from build123d import *

# Parameters (mm, degrees)
F0_R     = 1.4224
F1_DEPTH = 2.9718


with BuildPart() as f1:
    # F0 (on Front) → F1 (new body)
    with BuildSketch(Plane.XZ):
        Polygon((0, 25.4), (0, 0), (50.8, 0), (50.8, 11.2776), (45.72, 11.2776), (45.72, 8.1026), (42.545, 8.1026), (42.545, 11.2776), (36.957, 11.2776), (36.957, 14.1224), (42.545, 14.1224), (42.545, 17.2974), (45.72, 17.2974), (45.72, 14.1224), (50.8, 14.1224), (50.8, 25.4), align=None)
        with Locations((1.4859, 12.7)):
            Circle(F0_R, mode=Mode.SUBTRACT)
    extrude(amount=F1_DEPTH)


solid = f1.part
Build history of the part. All positions in model axes, mm. A direction names the side the tool comes from. Coordinates: 2 decimals unless noted, no trailing zeros. Order: outer loops, then holes, each group sorted by start corner. A loop starts at its lowest first (then second) coordinate and runs counter-clockwise, first axis right, second up. Notation, with made-up numbers: (27, -16.5) -> (66, -16.5) arc R34 cw to (66, 21.5) -> close; hole circle Ø11 at (47, 3.5). An arc over 180 degrees is marked (long way). One line per item, written item: value.
(1) Slice it at C-C, the plane z = 10.75. List the corners of the cut face in (x, y) (3 decimals), plus the area to 3 significant figures.
Checked values:
outline: (0, -2.972) -> (42.545, -2.972) -> (42.545, 0) -> (0, 0) -> close; (45.72, -2.972) -> (50.8, -2.972) -> (50.8, 0) -> (45.72, 0) -> close
area: 142 mm2
(2) Mould opens along Z. For faces 4 (the flat face through (25, -2.972, 13)), 5 (the flat face through (26, -1, 25.4)), 6 (the flat face through (48, -1, 11.278)) say: pulls with the +Z half, pulls with the -Z half, needs draft (parallel to the pull), parting line crosses it, or undercut.
Checked values:
face 4: needs draft
face 5: pulls with the +Z half
face 6: undercut
(3) Slice it at A-A, the plane y = -2.5. List the corners of the cut face in (x, z) (3 decimals).
Checked values:
outline: (0, 0) -> (50.8, 0) -> (50.8, 11.278) -> (45.72, 11.278) -> (45.72, 8.103) -> (42.545, 8.103) -> (42.545, 11.278) -> (36.957, 11.278) -> (36.957, 14.122) -> (42.545, 14.122) -> (42.545, 17.297) -> (45.72, 17.297) -> (45.72, 14.122) -> (50.8, 14.122) -> (50.8, 25.4) -> (0, 25.4) -> close; hole circle Ø2.845 at (1.486, 12.7)
(4) Slice it at B-B, the plane x = 39. List the corners of the cut face in (y, z), plus the area to 3 significant figures.
Checked values:
outline: (-2.97, 0) -> (0, 0) -> (0, 11.28) -> (-2.97, 11.28) -> close; (-2.97, 14.12) -> (0, 14.12) -> (0, 25.4) -> (-2.97, 25.4) -> close
area: 67.0 mm2
(5) Tool access for faces 1 (the flat face through (36.957, -1, 13)), 2 (the flat face through (50.8, -1, 6)), 3 (the flat face through (45.72, -1, 10)): list every direction of +Z, -Z, +X, -X, +Y, -Y with a clear straight run to the whole face (end or side of a thin tool).
Checked values:
face 1: +X, +Y, -Y
face 2: +Z, -Z, +X, +Y, -Y
face 3: +Y, -Y
(6) Probe line 1 (Z direction, x = 46, y = -1.1); line 2 (Z direction, x = 45.5, y = -1.05); line 3 (X direction, y = -2.4, z = 9.75) (3 decimals). List the from-to ranges inside material, lowest first. Write a range as [from, to].
Checked values:
line 1: [0, 11.28], [14.12, 25.4]
line 2: [0, 8.1], [17.3, 25.4]
line 3: [0, 42.545], [45.72, 50.8]
(7) Drop flat-ended pins along their axis: pin 1 Ø2.5 at (x, z) = (1.49, 12.7) entering from +Y; pin 2 Ø10 at (x, z) = (30.5, 8.5) entering from +Y. Give the stop position or say it passes through.
Checked values:
pin 1: through
pin 2: y = 0
